Verification items for the finished model (mm, model axes). Face numbers are marked on the shaded views. A direction names the side the tool comes from. Coordinates: 2 decimals unless noted, no trailing zeros. Write each loop counter-clockwise with the first axis right and the second up, starting at its lowest first coordinate (ties: lowest second). Pieces come first, ordered by that corner, then holes. Notation, with made-up numbers: (68, 53) -> (121, 53) arc R34 ccw to (121, 84) -> close; hole circle Ø8 at (-38, 9.5). An arc over 180 degrees is marked (long way). Use CSV: the item, a comma, the result in double quotes.
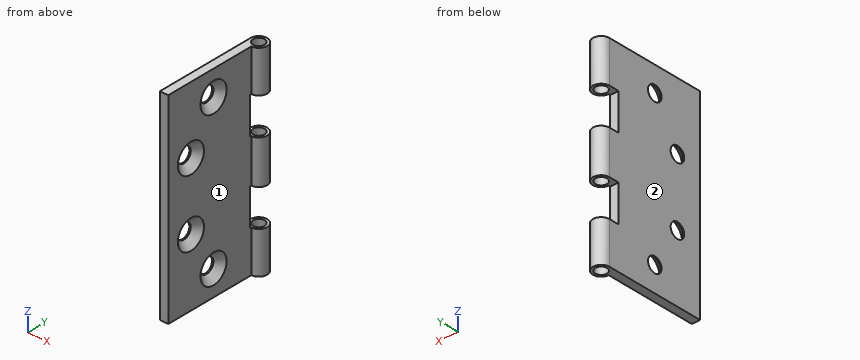
```python
from build123d import *

# Parameters (mm, degrees)
SKETCH_1_W                 = 5
SKETCH_1_H                 = 60
EXTRUDE_1_DEPTH            = 60
SKETCH_2_R                 = 5
SKETCH_4_R                 = 3.5
CUT_EXTRUDE_1_DEPTH        = 137.839321834
HOLE_WIZARD_M81_AT_2_COUNT = 2
HOLE_WIZARD_M81_AT_2_PITCH = 29.154759474
CUT_EXTRUDE_3_DEPTH        = 89.600225733
CUT_EXTRUDE_3_DEPTH_BACK   = 89.600225733
SKETCH_8_W                 = 22
SKETCH_8_H                 = 11


with BuildPart() as part:
    # Эскиз1 → Вытянуть-Тонкостенный1 (new, symmetric)
    with BuildSketch(Plane.XY):
        with Locations((2.5, 30)):
            Rectangle(SKETCH_1_W, SKETCH_1_H)
    extrude(amount=EXTRUDE_1_DEPTH, both=True)

    # По траектории1: sweep along a curve in space
    with BuildLine() as sweep_1_path:
        Line((5, 60, 60), (5, 60, -60))
    # Эскиз2 → По траектории1 (sweep)
    with BuildSketch(Plane.XY.offset(60)):
        with Locations((5, 60)):
            Circle(SKETCH_2_R)
    sweep(path=sweep_1_path.line)

    # Эскиз4 → Вырез-Вытянуть1 (cut, through all)
    with BuildSketch(Plane.XY.offset(60)):
        with Locations((5, 60)):
            Circle(SKETCH_4_R)
    extrude(amount=-CUT_EXTRUDE_1_DEPTH, mode=Mode.SUBTRACT)

    # Эскиз5 → Зенковка для  винта с плоской головкой M81 (revolve, cut)
    with BuildSketch(Plane(origin=(5, 30, 45), x_dir=(0, 0, -1), z_dir=(0, 1, 0))):
        Polygon((0, 0), (0, 5), (4.5, 5), (4.5, 4.15), (8.65, 0), align=None)
    hole_wizard_m81 = revolve(axis=Axis((11.35, 30, 45), (-1, 0, 0)), mode=Mode.SUBTRACT)

    # Зенковка для  винта с плоской головкой M81 at 2: Зенковка для  винта с плоской головкой M81 ×2
    with Locations(*[Vector(0, -0.5144957554275265, -0.8574929257125442) * (i * HOLE_WIZARD_M81_AT_2_PITCH) for i in range(1, HOLE_WIZARD_M81_AT_2_COUNT)]):
        add(hole_wizard_m81, mode=Mode.SUBTRACT)

    # Зеркальное отражение1: Зенковка для  винта с плоской головкой M81 across plane
    add(hole_wizard_m81.mirror(Plane.XY), mode=Mode.SUBTRACT)

    # Зеркальное отражение1 copy 1 sketch → Зеркальное отражение1 copy 1 (revolve, cut)
    with BuildSketch(Plane(origin=(5, 15, -20), x_dir=(0, 0, 1), z_dir=(0, 1, 0))):
        Polygon((0, 0), (0, -5), (4.5, -5), (4.5, -4.15), (8.65, 0), align=None)
    revolve(axis=Axis((11.35, 15, -20), (1, 0, 0)), mode=Mode.SUBTRACT)

    # Эскиз8 → Вырез-Вытянуть3 (cut, two sides: drawn at the far end of the back side and taken through both)
    with BuildSketch(Plane(origin=(5, 0, 0), x_dir=(0, 0, -1), z_dir=(1, 0, 0)).offset(-CUT_EXTRUDE_3_DEPTH_BACK)):
        with Locations((-24, 59.5)):
            Rectangle(SKETCH_8_W, SKETCH_8_H)
        with Locations((24, 59.5)):
            Rectangle(SKETCH_8_W, SKETCH_8_H)
    extrude(amount=CUT_EXTRUDE_3_DEPTH + CUT_EXTRUDE_3_DEPTH_BACK, mode=Mode.SUBTRACT)


solid = part.part
```
1) Scan lines: L1, parallel to Z at x = 0.25, y = 30; L2, parallel to Z at x = 1.5, y = 14; L3, parallel to X at y = 51, z = 9. Record each from-to range of solid material in increasing order.
Return value:
L1,"-60 to -49.5, -40.5 to 40.5, 49.5 to 60"
L2,"-60 to -25.05, -14.95 to 14.95, 25.05 to 60"
L3,"0 to 5"
2) Gauge pin test, flat ends, axial feed: pin 1 (8 mm diameter, centred on y = 14, z = -13.5, fed in from -X); pin 2 (2 mm diameter, centred on y = 44, z = -24.5, fed in from +X); pin 3 (11.5 mm diameter, centred on y = 30, z = 45, fed in from +X); pin 4 (1.5 mm diameter, centred on x = 1.5, z = 26.5, fed in from +Y). Record the tip position at first contact, or that the pin passes through.
Return value:
pin 1,"x = 0"
pin 2,"x = 5"
pin 3,"x = 2.1"
pin 4,"y = 54"
3) Cross-section at A-A (y = 30). Record the boundary of the cut face in (x, z), plus the area to 3 significant figures.
Return value:
outline,"(0, -60) -> (5, -60) -> (5, -53.65) -> (0.85, -49.5) -> (0, -49.5) -> close; (0, -40.5) -> (0.85, -40.5) -> (5, -36.35) -> (5, 36.35) -> (0.85, 40.5) -> (0, 40.5) -> close; (0, 49.5) -> (0.85, 49.5) -> (5, 53.65) -> (5, 60) -> (0, 60) -> close"
area,"476 mm2"
4) Cross-section at C-C (x = 3.5). Record the boundary of the cut face in (y, z).
Return value:
outline,"(0, -60) -> (56.84, -60) -> (56.84, -35) -> (54, -35) -> (54, -13) -> (56.84, -13) -> (56.84, 13) -> (54, 13) -> (54, 35) -> (56.84, 35) -> (56.84, 60) -> (0, 60) -> close; (63.16, -60) -> (64.77, -60) -> (64.77, -35) -> (63.16, -35) -> close; (63.16, -13) -> (64.77, -13) -> (64.77, 13) -> (63.16, 13) -> close; (63.16, 35) -> (64.77, 35) -> (64.77, 60) -> (63.16, 60) -> close; hole circle Ø14.3 at (15, -20); hole circle Ø14.3 at (15, 20); hole circle Ø14.3 at (30, -45); hole circle Ø14.3 at (30, 45)"
5) Cross-section at D-D (z = 20). Record the boundary of the cut face in (x, y), plus the area to 3 significant figures.
Return value:
outline,"(0, 0) -> (5, 0) -> (5, 6.35) -> (0.85, 10.5) -> (0, 10.5) -> close; (0, 19.5) -> (0.85, 19.5) -> (5, 23.65) -> (5, 54) -> (0, 54) -> close"
area,"208 mm2"
6) Set-up check for the marked faces 1 and 2: record each of +Z, -Z, +X, -X, +Y, -Y from which the full face is reachable in a straight line by a thin tool's end or side.
Return value:
face 1,"+Z, -Z, +X, -Y"
face 2,"+Z, -Z, -X, +Y, -Y"
7) Cross-section at B-B (z = 45). Record the boundary of the cut face in (x, y), plus the area to 3 significant figures.
Return value:
outline,"(0, 0) -> (5, 0) -> (5, 21.35) -> (0.85, 25.5) -> (0, 25.5) -> close; (0, 34.5) -> (0.85, 34.5) -> (5, 38.65) -> (5, 55) arc R5 ccw (long way) to (0, 60) -> close; hole circle Ø7 at (5, 60)"
area,"258 mm2"
